Could you check a few things on this model? Use its own coordinates, in mm. A direction names the side the tool comes from. Coordinates: 2 decimals unless noted, no trailing zeros. Loops run counter-clockwise (first coordinate to the right, second up) from the corner with the lowest first, then second, coordinate; pieces in that order, holes last. Notation, with made-up numbers: (89.5, 30) -> (118.5, 30) arc R32 ccw to (118.5, 66) -> close; hole circle Ø5 at (89.5, 67). An arc over 180 degrees is marked (long way). One line per question, with ' | ' between items.
```python
from build123d import *

# Parameters (mm, degrees)
F1_DEPTH = 25.4
F2_DEPTH = 44.45


with BuildPart() as f1:
    # F0 (on Front) → F1 (new body)
    with BuildSketch(Plane.XZ):
        with BuildLine():
            ThreePointArc((-39.6875, 49.3794158101), (-55.8319208878, 34.0674673207), (-77.3744968308, 28.4983099266))
            Line((-77.3744968308, 28.4983099266), (-54.2009934255, 28.4983099266))
            ThreePointArc((-54.2009934255, 28.4983099266), (-31.9759934255, 6.2733099266), (-54.2009934255, -15.9516900734))
            Line((-54.2009934255, -15.9516900734), (-77.3744968308, -15.9516900734))
            Line((-77.3744968308, -15.9516900734), (0, -38.6990942061))
            ThreePointArc((0, -38.6990942061), (12.4529146016, -36.068931174), (17.1085186303, -24.2233332247))
            ThreePointArc((17.1085186303, -24.2233332247), (26.2935862442, -17.2988786691), (37.5749282539, -19.544955343))
            ThreePointArc((37.5749282539, -19.544955343), (55.3627118113, -24.8347783768), (71.1983144283, -15.1589754969))
            ThreePointArc((71.1983144283, -15.1589754969), (75.0092778843, 22.014859432), (58.0413416028, 55.3091019392))
            ThreePointArc((58.0413416028, 55.3091019392), (41.3447910775, 59.999957233), (27.6341009885, 49.3794158101))
            ThreePointArc((27.6341009885, 49.3794158101), (14.6108004943, 40.0533008844), (1.5875, 49.3794158101))
            ThreePointArc((1.5875, 49.3794158101), (-4.4570838033, 34.7864996134), (-19.05, 28.7419158101))
            ThreePointArc((-19.05, 28.7419158101), (-33.6429161967, 34.7864996134), (-39.6875, 49.3794158101))
        make_face()
        with BuildLine():
            Line((44.0335609019, 0), (22.225, 0))
            ThreePointArc((22.225, 0), (-20.884668497, -7.6013976854), (17.0253377483, 14.2859546253))
            Line((17.0253377483, 14.2859546253), (37.8725077884, 31.778807317))
            ThreePointArc((37.8725077884, 31.778807317), (39.1080816416, 45.9014810832), (53.2307554079, 44.66590723))
            ThreePointArc((53.2307554079, 44.66590723), (62.7513822269, 23.341485137), (63.4919119209, 0))
            ThreePointArc((63.4919119209, 0), (53.7627364114, -9.7291755095), (44.0335609019, 0))
        make_face(mode=Mode.SUBTRACT)
        with BuildLine():
            ThreePointArc((17.0253377483, 14.2859546253), (20.884668497, 7.6013976854), (22.225, 0))
            Line((22.225, 0), (44.0335609019, 0))
            ThreePointArc((44.0335609019, 0), (43.9151265207, 16.4636733924), (37.8725077884, 31.778807317))
            Line((37.8725077884, 31.778807317), (17.0253377483, 14.2859546253))
        make_face()
    extrude(amount=F1_DEPTH)

    # F0 (on Front) → F2 (join)
    with BuildSketch(Plane.XZ):
        with BuildLine():
            ThreePointArc((-19.05, 70.0169158101), (-33.6429161967, 63.9723320068), (-39.6875, 49.3794158101))
            ThreePointArc((-39.6875, 49.3794158101), (-33.6429161967, 34.7864996134), (-19.05, 28.7419158101))
            Line((-19.05, 28.7419158101), (-19.05, 39.8544158101))
            ThreePointArc((-19.05, 39.8544158101), (-28.575, 49.3794158101), (-19.05, 58.9044158101))
            Line((-19.05, 58.9044158101), (-19.05, 70.0169158101))
        make_face()
        with BuildLine():
            ThreePointArc((1.5875, 49.3794158101), (-4.4570838033, 63.9723320068), (-19.05, 70.0169158101))
            Line((-19.05, 70.0169158101), (-19.05, 58.9044158101))
            ThreePointArc((-19.05, 58.9044158101), (-12.3148079092, 56.1146079009), (-9.525, 49.3794158101))
            Line((-9.525, 49.3794158101), (1.5875, 49.3794158101))
        make_face()
        with BuildLine():
            Line((-19.05, 39.8544158101), (-19.05, 28.7419158101))
            ThreePointArc((-19.05, 28.7419158101), (-4.4570838033, 34.7864996134), (1.5875, 49.3794158101))
            Line((1.5875, 49.3794158101), (-9.525, 49.3794158101))
            ThreePointArc((-9.525, 49.3794158101), (-12.3148079092, 42.6442237193), (-19.05, 39.8544158101))
        make_face()
        with BuildLine():
            Line((-54.2009934255, 28.4983099266), (-77.3744968308, 28.4983099266))
            ThreePointArc((-77.3744968308, 28.4983099266), (-99.5994968308, 6.2733099266), (-77.3744968308, -15.9516900734))
            Line((-77.3744968308, -15.9516900734), (-54.2009934255, -15.9516900734))
            ThreePointArc((-54.2009934255, -15.9516900734), (-31.9759934255, 6.2733099266), (-54.2009934255, 28.4983099266))
        make_face()
        with BuildLine():
            ThreePointArc((-77.3744968308, -8.0141900734), (-91.6619968308, 6.2733099266), (-77.3744968308, 20.5608099266))
            Line((-77.3744968308, 20.5608099266), (-54.2009934255, 20.5608099266))
            ThreePointArc((-54.2009934255, 20.5608099266), (-39.9668250993, 6.2733099266), (-54.2009934255, -8.0141900734))
            Line((-54.2009934255, -8.0141900734), (-77.3744968308, -8.0141900734))
        make_face(mode=Mode.SUBTRACT)
        with BuildLine():
            Line((22.225, 0), (14.2875, 0))
            ThreePointArc((14.2875, 0), (-13.4258583195, -4.8866127978), (10.9448599811, 9.1838279734))
            Line((10.9448599811, 9.1838279734), (17.0253377483, 14.2859546253))
            ThreePointArc((17.0253377483, 14.2859546253), (-20.884668497, -7.6013976854), (22.225, 0))
        make_face()
        with BuildLine():
            ThreePointArc((10.9448599811, 9.1838279734), (13.4258583195, 4.8866127978), (14.2875, 0))
            Line((14.2875, 0), (22.225, 0))
            ThreePointArc((22.225, 0), (20.884668497, 7.6013976854), (17.0253377483, 14.2859546253))
            Line((17.0253377483, 14.2859546253), (10.9448599811, 9.1838279734))
        make_face()
    extrude(amount=F2_DEPTH)


solid = f1.part
```
Q1. Please list where these lines run through material, in increasing order: L1, parallel to Z at x = 0, y = -33 (1 decimal); L2, parallel to Z at x = -19.05, y = -30; L3, parallel to X at y = -7.5, z = 15. Write a range as [from, to].
Values follow:
L1: z = [-22.2, -14.3], [14.3, 22.2], [41.4, 57.3] | L2: z = [-11.45, 11.45], [28.74, 39.85], [58.9, 70.02] | L3: x = [-97.81, -88.69], [-42.94, 44.17], [64.06, 75.93]
Q2. For pin 1 (10 mm diameter, centred on y = -31.5, z = -3, fed in from +X) (3 decimals); pin 2 (5 mm diameter, centred on y = -20, z = 21.5, fed in from +X); pin 3 (17 mm diameter, centred on x = 0, z = 0, fed in from +Y) (3 decimals); pin 4 (10 mm diameter, centred on x = 39.5, z = 22.5, fed in from +Y), each with a flat end and sliding along its axis, tell me the tip position at first contact or that it passes through.
Values follow:
pin 1: stops at x = 22.225 | pin 2: stops at x = 75.5 | pin 3: passes through | pin 4: stops at y = 0
Q3. We'd pull the mould along Z, two halves only. Please class faces 1 (the face through (-13, 0, 16)), 2 (the face through (43.959, -12.522, 16.236)), 3 (the face through (-66, -35, -15.952)): released by +Z, released by -Z, zero draft, split by the parting line, or undercut.
Values follow:
face 1: zero draft | face 2: undercut | face 3: released by -Z
Q4. Imagine slicing it at A-A on y = -30.5. Give the number of separate pieces and of enclosed holes in the cut face, plus the area to 3 significant figures.
Values follow:
separate pieces: 3 | enclosed holes: 3 | area: 3,240 mm2
Q5. Imagine slicing it at B-B on x = -84.5. Write out the boundary of the cut face in (y, z), plus the area to 3 significant figures.
Values follow:
outline: (-44.45, -14.78) -> (0, -14.78) -> (0, -6.11) -> (-44.45, -6.11) -> close; (-44.45, 18.66) -> (0, 18.66) -> (0, 27.33) -> (-44.45, 27.33) -> close | area: 771 mm2
Q6. Imagine slicing it at C-C on z = 37.5. Write out the boundary of the cut face in (x, y).
Values follow:
outline: (-50.56, -25.4) -> (-35.93, -25.4) -> (-35.93, -44.45) -> (-2.17, -44.45) -> (-2.17, -25.4) -> (35.55, -25.4) -> (35.55, 0) -> (-50.56, 0) -> close; (57.57, -25.4) -> (70.09, -25.4) -> (70.09, 0) -> (57.57, 0) -> close
Q7. Imagine slicing it at D-D on x = -34.5. Write out the boundary of the cut face in (y, z), plus the area to 3 significant figures.
Values follow:
outline: (-44.45, -4.01) -> (-25.4, -4.01) -> (-25.4, -28.56) -> (0, -28.56) -> (0, 63.06) -> (-44.45, 63.06) -> (-44.45, 35.7) -> (-25.4, 35.7) -> (-25.4, 16.56) -> (-44.45, 16.56) -> close | area: 3,240 mm2
Q8. For faces 4 (the face through (-31.98, -34.79, 5.78)), 5 (the face through (-66, -35, 28.498)), 6 (the face through (-91.66, -21.91, 5.96)), which set-ups out of +Z, -Z, +X, -X, +Y, -Y let a thin tool reach every point of the face, with its end or its side?
Values follow:
face 4: -Y | face 5: +Z, +X, -X, -Y | face 6: +Y, -Y
